Verification items for this drawing (mm, ordinates from the low corner). Round coordinates to 2 decimals unless told otherwise and drop trailing zeros. Order: outer loops, then holes, each group sorted by start corner. A loop starts at its lowest first (then second) coordinate and runs counter-clockwise, first axis right, second up.
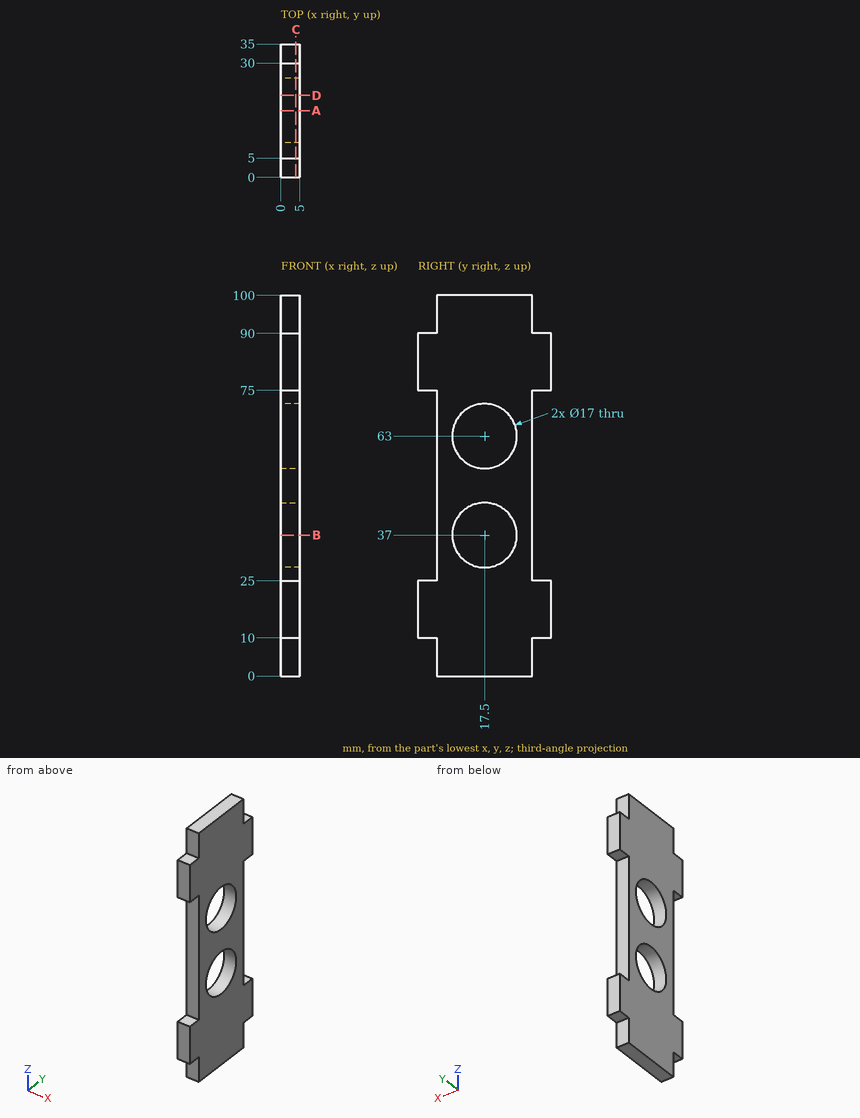
Item 1: Sectioned sample at C-C (x = 3.95). Record the cut outline in (y, z), and give its area (3 significant figures).
Answer:
outline: (0, 10) - (5, 10) - (5, 0) - (30, 0) - (30, 10) - (35, 10) - (35, 25) - (30, 25) - (30, 75) - (35, 75) - (35, 90) - (30, 90) - (30, 100) - (5, 100) - (5, 90) - (0, 90) - (0, 75) - (5, 75) - (5, 25) - (0, 25) - close; hole circle Ø17 at (17.5, 37); hole circle Ø17 at (17.5, 63)
area: 2,350 mm2
Item 2: Sectioned sample at B-B (z = 37). Record the cut outline in (x, y), and give its area (3 significant figures).
Answer:
outline: (0, 5) - (5, 5) - (5, 9) - (0, 9) - close; (0, 26) - (5, 26) - (5, 30) - (0, 30) - close
area: 40.0 mm2
Item 3: Sectioned sample at D-D (y = 21.5). Record the cut outline in (x, z).
Answer:
outline: (0, 0) - (5, 0) - (5, 29.5) - (0, 29.5) - close; (0, 44.5) - (5, 44.5) - (5, 55.5) - (0, 55.5) - close; (0, 70.5) - (5, 70.5) - (5, 100) - (0, 100) - close
Item 4: Sectioned sample at A-A (y = 17.5). Record the cut outline in (x, z), and give its area (3 significant figures).
Answer:
outline: (0, 0) - (5, 0) - (5, 28.5) - (0, 28.5) - close; (0, 45.5) - (5, 45.5) - (5, 54.5) - (0, 54.5) - close; (0, 71.5) - (5, 71.5) - (5, 100) - (0, 100) - close
area: 330 mm2
Item 5: Go/stop test with flat-tipped pins: P1, Ø2.5, axis at x = 2.5, z = 96, coming from the +Y side; P2, Ø2.5, axis at x = 3.5, y = 33, coming from the -Z side. Record where each tip stops, or that it passes through.
Answer:
P1: stops at y = 30
P2: stops at z = 10
Item 6: Scan lines: line 1 along Y through (x, z) = (3.5, 63); line 2 along Z through (x, y) = (3.7, 21.5); line 3 along Z through (x, y) = (2.7, 12). Record each from-to range of solid material in increasing order.
Answer:
line 1: y = 5 to 9, 26 to 30
line 2: z = 0 to 29.5, 44.5 to 55.5, 70.5 to 100
line 3: z = 0 to 30.52, 43.48 to 56.52, 69.48 to 100
